Part print with two shaded views. Sizes in mm from the minimum x, y, z corner. Round coordinates to 2 decimals unless told otherwise and drop trailing zeros. Write each loop counter-clockwise with the first axis right and the second up, starting at its lowest first coordinate (ties: lowest second). Pieces come first, ordered by that corner, then holes. Notation, with made-up numbers: (28, 62.5) -> (32, 62.5) arc R14 cw to (32, 72.5) -> close; hole circle Ø2 at (-16.5, 35.25). An arc over 180 degrees is marked (long way). Put each result on its own line as item: value. Start each with the question number.
1. Drill centre lines: line 1 (Y direction, x = 102.5, z = 3.9); line 2 (Y direction, x = 17, z = 4.8); line 3 (X direction, y = 28, z = 2.2) (1 decimal). Where is each one in solid material? Low to high. Write a range as from..to.
2. Saw through at B-B on x = 200. List the corners of the cut face in (y, z).
3. Saw through at C-C on y = 44. List the corners of the cut face in (x, z).
4. Saw through at A-A on z = 2.15. List the corners of the cut face in (x, y) (1 decimal), and give its area (3 significant figures).
5. Flat gauge pins, fed straight in: P1, Ø1.5, axis at x = 90.5, z = 2.5, coming from the +Y side; P2, Ø1.5, axis at x = 157, z = 2, coming from the +Y side (1 decimal); P3, Ø1.5, axis at y = 89, z = 3.5, coming from the +X side. Where does each tip first touch, or does it go through?
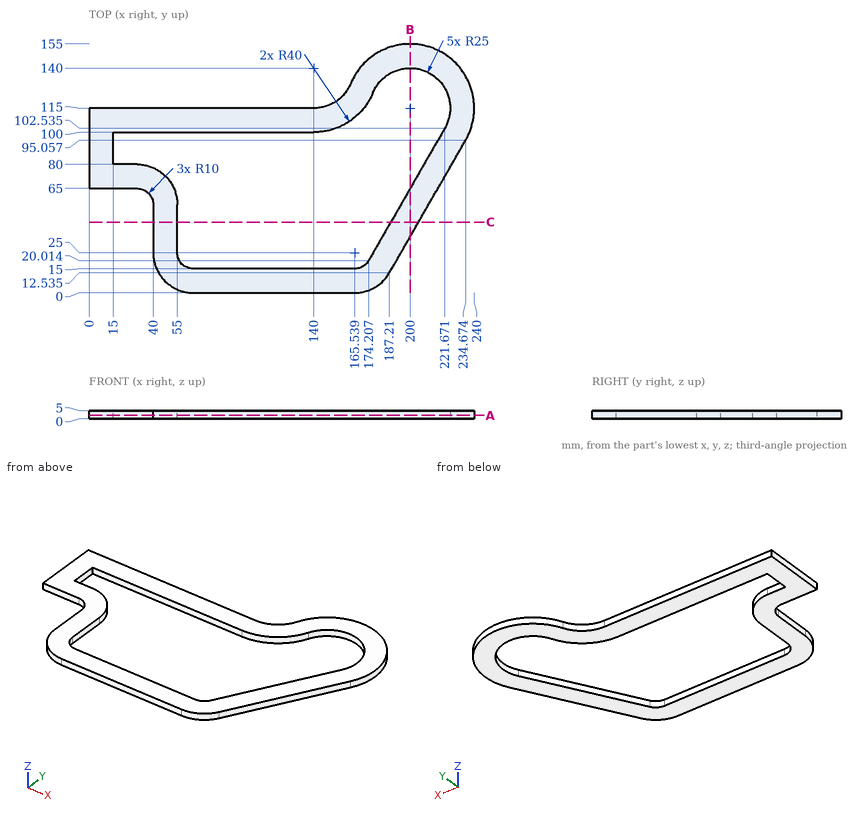
Return value:
1. line 1: y = 0..15, 100..115
1. line 2: y = 65..80, 100..115
1. line 3: x = 40..55, 178.8..196.1
2. outline: (34.77, 0) -> (64.86, 0) -> (64.86, 5) -> (34.77, 5) -> close; (140, 0) -> (155, 0) -> (155, 5) -> (140, 5) -> close
3. outline: (40, 0) -> (55, 0) -> (55, 5) -> (40, 5) -> close; (188, 0) -> (205.31, 0) -> (205.31, 5) -> (188, 5) -> close
4. outline: (0, 65) -> (30, 65) arc R10 cw to (40, 55) -> (40, 25) arc R25 ccw to (65, 0) -> (165.5, 0) arc R25 ccw to (187.2, 12.5) -> (234.7, 95.1) arc R40 ccw (long way) to (163.1, 130.4) arc R25 cw to (140, 115) -> (0, 115) -> close; hole (15, 80) -> (30, 80) arc R25 cw to (55, 55) -> (55, 25) arc R10 ccw to (65, 15) -> (165.5, 15) arc R10 ccw to (174.2, 20) -> (221.7, 102.5) arc R25 ccw (long way) to (176.9, 124.6) arc R40 cw to (140, 100) -> (15, 100) -> close
4. area: 9,500 mm^2
5. P1: stops at y = 115
5. P2: stops at y = 122.4
5. P3: stops at x = 231.62
